```python
from build123d import *

# Parameters (mm, degrees)
F0_W           = 180
F0_H           = 88
F1_DEPTH       = 20
F1_DEPTH_BACK  = 2
F2_R           = 5
F3_T           = -1.5
F4_W           = 6.8738348782
F4_H           = 1.2783666607
F5_DEPTH       = 90
F5_DEPTH_BACK  = 90
F6_R           = 1.75
F6_R_2         = 1
F7_DEPTH       = 90
F7_DEPTH_BACK  = 90
F8_W           = 5.3282827139
F8_H           = 1.7101019621
F9_DEPTH       = 90
F9_DEPTH_BACK  = 90
F10_DEPTH      = 80
F10_DEPTH_BACK = 80
F11_W          = 0.6596548483
F11_H          = 17.3489500303
F11_W_2        = 0.7256204262
F11_H_2        = 17.4149160739
F12_DEPTH      = 55.1
F13_DEPTH      = 4.3
F15_DEPTH      = 11.43
F15_DEPTH_BACK = 10.21


with BuildPart() as f1:
    # F0 (on Top) → F1 (new body, two sides)
    with BuildSketch(Plane.XY) as f1_sk:
        Rectangle(F0_W, F0_H)
    extrude(amount=F1_DEPTH)
    extrude(f1_sk.sketch, amount=-F1_DEPTH_BACK)

    # F2
    f2_edges = [f1.edges().sort_by_distance(p)[0] for p in [
        (0, -44, 20),
        (90, 0, 20),
        (0, 44, 20),
        (-90, 0, 20),
    ]]
    fillet(f2_edges, radius=F2_R)

    # F3
    f3_openings = [f1.faces().sort_by_distance(p)[0] for p in [
        (0, 0, -2),
    ]]
    offset(amount=F3_T, openings=f3_openings)

    # F4 (on Right) → F5 (join, two sides)
    with BuildSketch(Plane.YZ) as f5_sk:
        with Locations((-47.1954066306, 0.6391833303)):
            Rectangle(F4_W, F4_H)
    extrude(amount=F5_DEPTH)
    extrude(f5_sk.sketch, amount=-F5_DEPTH_BACK)

    # F6 (on Right) → F7 (join, two sides)
    with BuildSketch(Plane.YZ) as f7_sk:
        with Locations((-51.9656985998, 0.5429131561)):
            Circle(F6_R)
        with Locations((-51.9656985998, 0.5429131561)):
            Circle(F6_R_2, mode=Mode.SUBTRACT)
    extrude(amount=F7_DEPTH)
    extrude(f7_sk.sketch, amount=-F7_DEPTH_BACK)

    # F8 (on Right) → F9 (cut, two sides)
    with BuildSketch(Plane.YZ) as f9_sk:
        with Locations((-52.9466792941, -0.855050981)):
            Rectangle(F8_W, F8_H)
    extrude(amount=F9_DEPTH, mode=Mode.SUBTRACT)
    extrude(f9_sk.sketch, amount=-F9_DEPTH_BACK, mode=Mode.SUBTRACT)

    # F8 (on Right) → F10 (cut, two sides)
    with BuildSketch(Plane.YZ) as f10_sk:
        with Locations((-52.9466792941, -0.855050981)):
            Rectangle(F8_W, F8_H)
    extrude(amount=-F10_DEPTH, mode=Mode.SUBTRACT)
    extrude(f10_sk.sketch, amount=F10_DEPTH_BACK, mode=Mode.SUBTRACT)

    # F11 (on Front) → F12 (cut)
    with BuildSketch(Plane.XZ):
        with Locations((11.7518459447, 4.9456743291)):
            Rectangle(F11_W, F11_H)
        with Locations((-10.5775059201, 4.9126913073)):
            Rectangle(F11_W_2, F11_H_2)
    extrude(amount=-F12_DEPTH, mode=Mode.SUBTRACT)

    # F13 (add): a face of the model
    f13_faces = [f1.faces().sort_by_distance(p)[0] for p in [
        (0.6036614068, 43.25, -2),
    ]]
    extrude(f13_faces, amount=F13_DEPTH)

    # F14 (on Right) → F15 (join, two sides)
    with BuildSketch(Plane.YZ) as f15_sk:
        Polygon((43.986722827, -6.3001378439), (44.0000370145, -6.2996791676), (44.851500541, -5.855040258), (44.851500541, -5.530836992), (43.986722827, -5.530836992), align=None)
    extrude(amount=F15_DEPTH)
    extrude(f15_sk.sketch, amount=-F15_DEPTH_BACK)


solid = f1.part
```
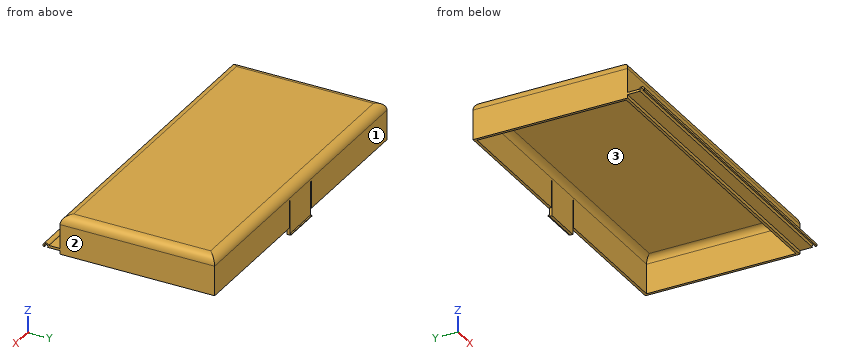
Check sheet for the modelled part. Datum: model origin and axes. Units: mm. Face numbers are marked on the shaded views. A direction names the side the tool comes from. Coordinates: 2 decimals unless noted, no trailing zeros. Loops run counter-clockwise (first coordinate to the right, second up) from the corner with the lowest first, then second, coordinate; pieces in that order, holes last.
1) Sectioned sample at A-A (z = 10). Record the boundary of the cut face in (x, y).
2) Access from +Z, -Z, +X, -X, +Y, -Y to the whole of each face (thin tool, end or side, straight path). Record for the marked faces 1, 2 and 3.
3) Sectioned sample at B-B (x = 42.5). Record the boundary of the cut face in (y, z).
4) Gauge pin test, flat ends, axial feed: pin 1 (8 mm diameter, centred on x = 64.5, z = 12, fed in from +Y); pin 2 (7 mm diameter, centred on x = 32, z = 11, fed in from -Y); pin 3 (6 mm diameter, centred on x = -43, y = -30, fed in from -Z); pin 4 (6 mm diameter, centred on y = -13.5, z = 17.5, fed in from -X). Record the tip position at first contact, or that the pin passes through.
5) Sectioned sample at C-C (y = 27). Record the boundary of the cut face in (x, z).
6) Material ranges on probe 1 along Y at (x, z) = (45.5, 0.5); probe 2 along Y at (x, z) = (-14, 13); probe 3 along X at (y, z) = (16, -1.25), recorded low to high.
Check sheet entries:
1. outline: (-90, -44) - (90, -44) - (90, 44) - (12.08, 44) - (12.08, 42.5) - (88.5, 42.5) - (88.5, -42.5) - (-88.5, -42.5) - (-88.5, 42.5) - (-10.94, 42.5) - (-10.94, 44) - (-90, 44) - close; (-10.21, 42.5) - (11.42, 42.5) - (11.42, 44) - (-10.21, 44) - close
2. face 1: +Z, +X, -X, +Y
2. face 2: +Z, -Z, +X, +Y, -Y
2. face 3: -Z
3. outline: (-53.63, 0) - (-52.81, 0) arc R1 cw (long way) to (-51.13, 0) - (-44, 0) - (-44, -2) - (-42.5, -2) - (-42.5, 15) arc R3.5 cw to (-39, 18.5) - (39, 18.5) arc R3.5 cw to (42.5, 15) - (42.5, -2) - (44, -2) - (44, 15) arc R5 ccw to (39, 20) - (-39, 20) arc R5 ccw to (-44, 15) - (-44, 1.28) - (-50.38, 1.28) arc R1.75 ccw to start
4. pin 1: stops at y = 44
4. pin 2: stops at y = -44
4. pin 3: stops at z = 18.5
4. pin 4: stops at x = -90
5. outline: (-90, -2) - (-88.5, -2) - (-88.5, 15) arc R3.5 cw to (-85, 18.5) - (85, 18.5) arc R3.5 cw to (88.5, 15) - (88.5, -2) - (90, -2) - (90, 15) arc R5 ccw to (85, 20) - (-85, 20) arc R5 ccw to (-90, 15) - close
6. probe 1: y = -53.72 to -52.96, -50.97 to -42.5, 42.5 to 44
6. probe 2: y = -44 to -42.5, 42.5 to 44
6. probe 3: x = -90 to -88.5, 88.5 to 90
